from build123d import *

# Parameters (mm, degrees)
SKIZZE3_R     = 1.5
SKIZZE3_R_2   = 0.5
ACHSE_1_DEPTH = 5
SKIZZE4_R     = 1.5
SKIZZE4_R_2   = 0.5
ACHSE_2_DEPTH = 5


with BuildPart() as part:
    # Skizze2 → Kugel (revolve)
    with BuildSketch(Plane(origin=(0, 0, 0), x_dir=(0, 0, -1), z_dir=(1, 0, 0))):
        with BuildLine():
            Line((0, 6), (0, -6))
            ThreePointArc((0, -6), (6, 0), (0, 6))
        make_face()
    revolve(axis=Axis((0, 23.376095618, 0), (0, -1, 0)))

    # Skizze3 → Achse 1 (cut, symmetric)
    with BuildSketch(Plane(origin=(0, 0, 0), x_dir=(0, 0, -1), z_dir=(1, 0, 0))):
        Circle(SKIZZE3_R)
        with Locations((0, 2.5)):
            Circle(SKIZZE3_R_2)
    extrude(amount=ACHSE_1_DEPTH, both=True, mode=Mode.SUBTRACT)

    # Skizze4 → Achse 2 (cut, symmetric)
    with BuildSketch(Plane(origin=(0, 0, 0), x_dir=(1, 0, 0), z_dir=(0, 1, 0))):
        Circle(SKIZZE4_R)
        with Locations((0, 2.5)):
            Circle(SKIZZE4_R_2)
    extrude(amount=ACHSE_2_DEPTH, both=True, mode=Mode.SUBTRACT)


solid = part.part
CAD build for the part. Positions are in the model's coordinates, mm. Give positions to 0.01 mm unless a question says otherwise; leave off trailing zeros. Loops run counter-clockwise (first coordinate to the right, second up) from the corner with the lowest first, then second, coordinate; pieces in that order, holes last. Notation, with made-up numbers: M 42.25,17.5 L 88.25,17.5 A36 cw 88.25,53.5 Z; hole C 27.5,13 d1. An arc over 180 degrees is marked long. Write each question's results on one line, items separated by ' | '.
Q1. Band-saw the part on C-C on y = 2.5. Write the cut outline in (x, z).
Geometry check:
outline: C 0,0 d10.91; hole M -5,-0.5 L -1.41,-0.5 A1.5 ccw 1.41,-0.5 L 5,-0.5 L 5,0.5 L 1.41,0.5 A1.5 ccw -1.41,0.5 L -5,0.5 Z; hole C 0,-2.5 d1
Q2. Band-saw the part on D-D on z = 3. Write the cut outline in (x, y), and give its area (3 significant figures).
Geometry check:
outline: C 0,0 d10.39 | area: 84.8 mm²
Q3. Flat gauge pins, fed straight in: P1, Ø5, axis at x = -3, y = 3, coming from the +Z side; P2, Ø4, axis at x = 4.5, y = 4, coming from the -Z side; P3, Ø1, axis at x = 4, y = -4, coming from the +Z side. Where does each tip first touch, or does it go through?
Geometry check:
P1: stops at z = 5.74 | P2: stops at z = -4.45 | P3: stops at z = 3.07
Q4. Band-saw the part on B-B on x = -0.25. Write the cut outline in (y, z), and give its area (3 significant figures).
Geometry check:
outline: C 0,0 d11.99; hole M -5,-2.93 L 5,-2.93 L 5,-2.07 L -5,-2.07 Z; hole M -5,-1.48 L -0.25,-1.48 A1.5 ccw 0.25,-1.48 L 5,-1.48 L 5,1.48 L 0.25,1.48 A1.5 ccw -0.25,1.48 L -5,1.48 Z | area: 74.6 mm²
Q5. Probe probe 1 along Y at (x, z) = (3.2, 0); probe 2 along Z at (x, y) = (0, 3.8); probe 3 along Y at (x, z) = (4.2, 0). List the from-to ranges inside material, lowest first.
Geometry check:
probe 1: y = -5.08 to -1.5, 1.5 to 2, 3 to 5.08 | probe 2: z = -4.64 to -3, -2 to -1.5, 1.5 to 4.64 | probe 3: y = -4.28 to -1.5, 1.5 to 2, 3 to 4.28
Q6. Band-saw the part on A-A on z = 0. Write the cut outline in (x, y), and give its area (3 significant figures).
Geometry check:
outline: C 0,0 d12; hole M -5,-1.5 L -1.5,-1.5 L -1.5,-5 L 1.5,-5 L 1.5,-1.5 L 5,-1.5 L 5,1.5 L 1.5,1.5 L 1.5,2 L 5,2 L 5,3 L 1.5,3 L 1.5,5 L -1.5,5 L -1.5,3 L -5,3 L -5,2 L -1.5,2 L -1.5,1.5 L -5,1.5 Z | area: 55.1 mm²
